Model file for the job. Use its own axes, mm. A direction names the side the tool comes from. Coordinates: 2 decimals unless noted, no trailing zeros. Order: outer loops, then holes, each group sorted by start corner. A loop starts at its lowest first (then second) coordinate and runs counter-clockwise, first axis right, second up. Notation, with made-up numbers: (39, 77.5) -> (56, 77.5) arc R19 ccw to (56, 92.5) -> close; hole circle Ø6 at (56, 44.25). An arc over 180 degrees is marked (long way). Return JSON: item names as keys, results as strings. Group by question number.
1) Cut at D-D (z = 8.5). Write the cut outline in (x, y), and give its area (3 significant figures).
2) Cut at A-A (y = 17). Write the cut outline in (x, z).
3) Cut at B-B (x = 0). Write the cut outline in (y, z).
4) Flat gauge pins, fed straight in: pin 1 (5 mm diameter, centred on x = -2, y = -15.5, fed in from -Z); pin 2 (0.8 mm diameter, centred on y = -30, z = 17, fed in from +X); pin 3 (1.5 mm diameter, centred on y = -2, z = 4, fed in from +X); pin 4 (3 mm diameter, centred on y = -13, z = 3.5, fed in from -X). Where does each tip first touch, or does it go through?
5) Pull direction X, two halves, no side cores. Call faces 4 (the flat face through (26, 34, 13)), 5 (the flat face through (-26, 34, 13)), 6 (the cylindrical face through (-0.629, -16.488, 8.874)), 7 (the flat face through (-19.59, 46.1, 33.43)): +X half, -X half, draft (parallel to the pull), parting line (faces both ways), or undercut.
6) Which spindle directions (+Z, -Z, +X, -X, +Y, -Y) get a long thin tool onto all of the face, cutting with end or side? Do faces 1 (the flat face through (-6, -33, 17)), 2 (the flat face through (0, 55, 13)), 3 (the flat face through (-13, 45, 26)). Say none if no direction does.
7) Probe line 1 (X direction, y = 0, z = 10.25); line 2 (X direction, y = 17, z = 14.5); line 3 (Z direction, x = -11.5, y = -28.5). List the from-to ranges inside material, lowest first.
8) Cut at C-C (z = 29). Write the cut outline in (x, y).
from build123d import *

# Parameters (mm, degrees)
EXTRUDE_1_DEPTH     = 18
EXTRUDE_2_DEPTH     = 13
CUT_EXTRUDE_1_DEPTH = 2.5


with BuildPart() as part:
    # 草图1 → 凸台-拉伸1 (new body)
    with BuildSketch(Plane.XY):
        Polygon((-26, 0), (-15, -40), (15, -40), (26, 0), (26, 55), (-26, 55), align=None)
        with BuildLine():
            ThreePointArc((-6.727579547, 15.066176471), (0, -16.5), (6.727579547, 15.066176471))
            ThreePointArc((6.727579547, 15.066176471), (0, 24), (-6.727579547, 15.066176471))
        make_face(mode=Mode.SUBTRACT)
    extrude(amount=EXTRUDE_1_DEPTH)

    # 草图2 → 凸台-拉伸2 (add)
    with BuildSketch(Plane(origin=(26, 0, 0), x_dir=(0, 0, -1), z_dir=(1, 0, 0))):
        Polygon((-18, 55), (-18, 35), (-31.905808723, 37.451969267), (-35, 55), align=None)
    extrude_2 = extrude(amount=-EXTRUDE_2_DEPTH)

    # 镜向1: 凸台-拉伸2 across plane
    add(extrude_2.mirror(Plane(origin=(0, 0, 0), x_dir=(0, 0, 1), z_dir=(1, 0, 0))))

    # 草图3 → 切除-拉伸1 (cut, symmetric)
    with BuildSketch(Plane.XY.offset(18)):
        with BuildLine():
            Line((-6, -26), (-6, -55.48155058))
            Line((-6, -55.48155058), (6, -55.48155058))
            Line((6, -55.48155058), (6, -26))
            ThreePointArc((6, -26), (0, -20), (-6, -26))
        make_face()
    extrude(amount=CUT_EXTRUDE_1_DEPTH, both=True, mode=Mode.SUBTRACT)


solid = part.part
Answers below:
{
 "1": {"outline": "(-26, 0) -> (-15, -40) -> (15, -40) -> (26, 0) -> (26, 55) -> (-26, 55) -> close; hole (-6.73, 15.07) arc R16.5 ccw (long way) to (6.73, 15.07) arc R7 ccw (long way) to start", "area": "3,550 mm^2"},
 "2": {"outline": "(-26, 0) -> (-7, 0) -> (-7, 18) -> (-26, 18) -> close; (7, 0) -> (26, 0) -> (26, 18) -> (7, 18) -> close"},
 "3": {"outline": "(-40, 0) -> (-16.5, 0) -> (-16.5, 18) -> (-20, 18) -> (-20, 15.5) -> (-40, 15.5) -> close; (24, 0) -> (55, 0) -> (55, 18) -> (24, 18) -> close"},
 "4": {"pin 1": "stops at z = 0", "pin 2": "stops at x = 17.86", "pin 3": "stops at x = 25.66", "pin 4": "stops at x = -22.84"},
 "5": {"face 4": "+X half", "face 5": "-X half", "face 6": "undercut", "face 7": "draft"},
 "6": {"face 1": "+Z, -Y", "face 2": "+Z, -Z, +X, -X, +Y", "face 3": "+Z, +Y, -Y"},
 "7": {"line 1": "x = -26 to -16.5, 16.5 to 26", "line 2": "x = -26 to -7, 7 to 26", "line 3": "z = 0 to 18"},
 "8": {"outline": "(-26, 36.94) -> (-13, 36.94) -> (-13, 55) -> (-26, 55) -> close; (13, 36.94) -> (26, 36.94) -> (26, 55) -> (13, 55) -> close"}
}
